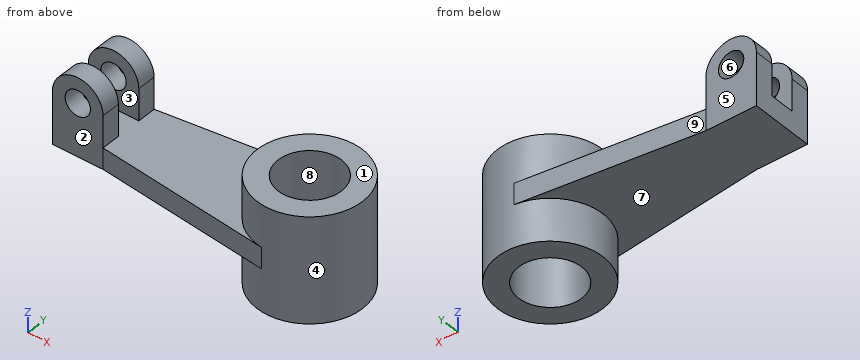
Solid Edge part; units mm, degrees
sketch "Sketch1" plane through (0, 0, 0) normal (0, 0, 1) x (1, 0, 0)
  circle A0 centre (0, 0) radius 25
extrude "Protrusion1" add sketch "Sketch1" along normal mid plane 50
sketch "Sketch2" plane through (0, 0, 0) normal (0, 0, 1) x (1, 0, 0)
  line L0 (-86, -15) -> (-2.9372, -24.8269)
  line L1 (-110, -15) -> (-86, -15)
  line L2 (-110, 15) -> (-110, -15)
  line L3 (-86, 15) -> (-110, 15)
  line L4 (-86, 15) -> (-2.9372, 24.8269)
extrude "ExtrudedProtrusion_2" add sketch "Sketch2" along normal mid plane 10 material side at (-44.4745, -19.9631, 0)
sketch "Sketch3" plane through (0, 0, 0) normal (0, 0, 1) x (1, 0, 0)
  circle A0 centre (0, 0) radius 15
extrude "Cutout1" cut sketch "Sketch3" along normal up to next and the other way up to next
sketch "Sketch4" plane through (-98, -15, 0) normal (0, -1, 0) x (1, 0, 0)
  line L0 (12, 5) -> (12, 20)
  line L1 (12, 5) -> (-12, 5)
  line L2 (-12, 5) -> (-12, 20)
  arc A0 (-12, 20) -> (12, 20) centre (0, 20) cw
extrude "ExtrudedProtrusion_3" add sketch "Sketch4" against normal blind 9
mirror "Mirror1" about plane through (0, 0, 0) normal (0, -1, 0) of "ExtrudedProtrusion_3"
sketch "Sketch5" plane through (-98, -15, 0) normal (0, -1, 0) x (1, 0, 0)
  circle A0 centre (0, 20) radius 6
extrude "Cutout2" cut sketch "Sketch5" against normal through all
Here's how the part is built. I have some questions about the finished solid (model axes, mm). Face numbers are marked on the shaded views. A direction names the side the tool comes from. Coordinates: 2 decimals unless noted, no trailing zeros. Order: outer loops, then holes, each group sorted by start corner. A loop starts at its lowest first (then second) coordinate and runs counter-clockwise, first axis right, second up.
Item 1: For P1, Ø4, axis at x = -12, z = -0.5, coming from the -Y side; P2, Ø10, axis at y = 12.5, z = 11.5, coming from the +X side; P3, Ø7, axis at x = -93.5, z = 14.5, coming from the +Y side; P4, Ø11, axis at x = -98, z = 20, coming from the +Y side, each with a flat end and sliding along its axis, tell me the tip position at first contact or that it passes through.
Result sheet:
P1: stops at y = -23.99
P2: stops at x = 23.85
P3: stops at y = 15
P4: passes through
Item 2: If we section it at C-C on y = -12: List the corners of the cut face in (x, z) for me, plus the area to 3 significant figures.
Result sheet:
outline: (-110, -5) - (-21.93, -5) - (-21.93, -25) - (-9, -25) - (-9, 25) - (-21.93, 25) - (-21.93, 5) - (-86, 5) - (-86, 20) arc R12 ccw to (-110, 20) - close; (9, -25) - (21.93, -25) - (21.93, 25) - (9, 25) - close; hole circle Ø12 at (-98, 20)
area: 2,650 mm2
Item 3: If we section it at B-B on x = -98: List the corners of the cut face in (y, z) for me.
Result sheet:
outline: (-15, -5) - (15, -5) - (15, 14) - (6, 14) - (6, 5) - (-6, 5) - (-6, 14) - (-15, 14) - close; (-15, 26) - (-6, 26) - (-6, 32) - (-15, 32) - close; (6, 26) - (15, 26) - (15, 32) - (6, 32) - close
Item 4: For the marked faces 1, 2, 3, 4 and 5, which set-ups out of +Z, -Z, +X, -X, +Y, -Y let a thin tool reach every point of the face, with its end or its side?
Result sheet:
face 1: +Z, +X, +Y, -Y
face 2: +Z, -Z, -X, -Y
face 3: +Z, -X
face 4: none
face 5: +Z, -Z, -X, +Y
Item 5: If we section it at A-A on y = 0: List the corners of the cut face in (x, z) for me.
Result sheet:
outline: (-110, -5) - (-25, -5) - (-25, -25) - (-15, -25) - (-15, 25) - (-25, 25) - (-25, 5) - (-110, 5) - close; (15, -25) - (25, -25) - (25, 25) - (15, 25) - close
Item 6: If we mould it in two halves opening along X, with no side actions, what happens to the marked faces 6, 7, 8 and 9? For each: +X half, -X half, draft (parallel to the pull), parting line (faces both ways), or undercut.
Result sheet:
face 6: undercut
face 7: draft
face 8: undercut
face 9: -X half
Item 7: I need wall thicknesses on line 1 (Y direction, x = 0, z = -15); line 2 (X direction, y = 0, z = -1); line 3 (Z direction, x = -98, y = 9.5). Which ranges of each line are inside material? Lowest first, please.
Result sheet:
line 1: y = -25 to -15, 15 to 25
line 2: x = -110 to -15, 15 to 25
line 3: z = -5 to 14, 26 to 32
